```python
from build123d import *

# Parameters (mm, degrees)
F1_DEPTH = 10
F2_START = 6.1
F2_DEPTH = 3.9


with BuildPart() as f1:
    # F0 (on Front) → F1 (new body)
    with BuildSketch(Plane.XZ):
        with BuildLine():
            ThreePointArc((-36.2228804372, 67.6292184035), (-37.698913152, 69.3123111398), (-39.8481115853, 69.9387453565))
            Line((-39.8481115853, 69.9387453565), (-154.2675887644, 69.9387453565))
            Line((-154.2675887644, 69.9387453565), (-174, 66.5009789131))
            Line((-174, 66.5009789131), (-165.0019578262, 27.5261763217))
            Line((-165.0019578262, 27.5261763217), (-149.4120367897, 31.1253931912))
            ThreePointArc((-149.4120367897, 31.1253931912), (-146.3925555154, 30.6201053167), (-144.6147523132, 28.1277171494))
            Line((-144.6147523132, 28.1277171494), (-132.5798709058, -24.0010813166))
            ThreePointArc((-132.5798709058, -24.0010813166), (-133.0851587803, -27.0205625909), (-135.5775469475, -28.7983657931))
            Line((-135.5775469475, -28.7983657931), (-151.1674679841, -32.3975826626))
            Line((-151.1674679841, -32.3975826626), (-142.1694258103, -71.372385254))
            Line((-142.1694258103, -71.372385254), (-122.6820245146, -66.8733641671))
            Line((-122.6820245146, -66.8733641671), (122.6820245146, -66.8733641671))
            Line((122.6820245146, -66.8733641671), (142.1694258103, -71.372385254))
            Line((142.1694258103, -71.372385254), (151.1674679841, -32.3975826626))
            Line((151.1674679841, -32.3975826626), (135.5775469475, -28.7983657931))
            ThreePointArc((135.5775469475, -28.7983657931), (133.0851587803, -27.0205625909), (132.5798709058, -24.0010813166))
            Line((132.5798709058, -24.0010813166), (144.6147523132, 28.1277171494))
            ThreePointArc((144.6147523132, 28.1277171494), (146.3925555154, 30.6201053167), (149.4120367897, 31.1253931912))
            Line((149.4120367897, 31.1253931912), (165.0019578262, 27.5261763217))
            Line((165.0019578262, 27.5261763217), (174, 66.5009789131))
            Line((174, 66.5009789131), (154.2675887644, 69.9387453565))
            Line((154.2675887644, 69.9387453565), (39.8481115853, 69.9387453565))
            ThreePointArc((39.8481115853, 69.9387453565), (37.698913152, 69.3123111398), (36.2228804372, 67.6292184035))
            Line((36.2228804372, 67.6292184035), (6.3441545093, 3.554083875))
            ThreePointArc((6.3441545093, 3.554083875), (0, -0.4875882928), (-6.3441545093, 3.554083875))
            Line((-6.3441545093, 3.554083875), (-36.2228804372, 67.6292184035))
        make_face()
        with BuildLine():
            Line((-96.7999833788, -41.9593826596), (-92.2684444436, -39.8462913509))
            Line((-92.2684444436, -39.8462913509), (-19.7638214806, -6.0368304117))
            Line((-19.7638214806, -6.0368304117), (-15.2322825455, -3.923739103))
            ThreePointArc((-15.2322825455, -3.923739103), (-1.8101294528, -8.8090033085), (-6.6953936583, -22.2311564011))
            Line((-6.6953936583, -22.2311564011), (-11.2269325935, -24.3442477098))
            Line((-11.2269325935, -24.3442477098), (-83.7315555564, -58.1537086491))
            Line((-83.7315555564, -58.1537086491), (-88.2630944916, -60.2667999578))
            ThreePointArc((-88.2630944916, -60.2667999578), (-101.6852475843, -55.3815357523), (-96.7999833788, -41.9593826596))
        make_face(mode=Mode.SUBTRACT)
        with BuildLine():
            Line((88.2630944916, -60.2667999578), (83.7315555564, -58.1537086491))
            Line((83.7315555564, -58.1537086491), (11.2269325935, -24.3442477098))
            Line((11.2269325935, -24.3442477098), (6.6953936583, -22.2311564011))
            ThreePointArc((6.6953936583, -22.2311564011), (1.8101294528, -8.8090033085), (15.2322825455, -3.923739103))
            Line((15.2322825455, -3.923739103), (19.7638214806, -6.0368304117))
            Line((19.7638214806, -6.0368304117), (92.2684444436, -39.8462913509))
            Line((92.2684444436, -39.8462913509), (96.7999833788, -41.9593826596))
            ThreePointArc((96.7999833788, -41.9593826596), (101.6852475843, -55.3815357523), (88.2630944916, -60.2667999578))
        make_face(mode=Mode.SUBTRACT)
        with BuildLine():
            ThreePointArc((-65.576829212, -14.2695895243), (-82.8528678461, -7.9816256954), (-76.5649040173, 9.2944129387))
            Line((-76.5649040173, 9.2944129387), (-67.5018261469, 13.5205955561))
            ThreePointArc((-67.5018261469, 13.5205955561), (-50.2257875128, 7.2326317272), (-56.5137513416, -10.0434069069))
            Line((-56.5137513416, -10.0434069069), (-65.576829212, -14.2695895243))
        make_face(mode=Mode.SUBTRACT)
        with BuildLine():
            Line((-40.8102109153, 39.0972973828), (-113.3148338783, 5.2878364435))
            Line((-113.3148338783, 5.2878364435), (-117.8463728135, 3.1747451348))
            ThreePointArc((-117.8463728135, 3.1747451348), (-131.2685259061, 8.0600093403), (-126.3832617006, 21.4821624329))
            Line((-126.3832617006, 21.4821624329), (-121.8517227654, 23.5952537416))
            Line((-121.8517227654, 23.5952537416), (-49.3470998025, 57.4047146809))
            Line((-49.3470998025, 57.4047146809), (-44.8155608673, 59.5178059896))
            ThreePointArc((-44.8155608673, 59.5178059896), (-31.3934077747, 54.6325417841), (-36.2786719802, 41.2103886915))
            Line((-36.2786719802, 41.2103886915), (-40.8102109153, 39.0972973828))
        make_face(mode=Mode.SUBTRACT)
        with BuildLine():
            ThreePointArc((76.5649040173, 9.2944129387), (82.8528678461, -7.9816256954), (65.576829212, -14.2695895243))
            Line((65.576829212, -14.2695895243), (56.5137513416, -10.0434069069))
            ThreePointArc((56.5137513416, -10.0434069069), (50.2257875128, 7.2326317272), (67.5018261469, 13.5205955561))
            Line((67.5018261469, 13.5205955561), (76.5649040173, 9.2944129387))
        make_face(mode=Mode.SUBTRACT)
        with BuildLine():
            Line((49.3470998025, 57.4047146809), (121.8517227654, 23.5952537416))
            Line((121.8517227654, 23.5952537416), (126.3832617006, 21.4821624329))
            ThreePointArc((126.3832617006, 21.4821624329), (131.2685259061, 8.0600093403), (117.8463728135, 3.1747451348))
            Line((117.8463728135, 3.1747451348), (113.3148338783, 5.2878364435))
            Line((113.3148338783, 5.2878364435), (40.8102109153, 39.0972973828))
            Line((40.8102109153, 39.0972973828), (36.2786719802, 41.2103886915))
            ThreePointArc((36.2786719802, 41.2103886915), (31.3934077747, 54.6325417841), (44.8155608673, 59.5178059896))
            Line((44.8155608673, 59.5178059896), (49.3470998025, 57.4047146809))
        make_face(mode=Mode.SUBTRACT)
    extrude(amount=F1_DEPTH)

    # F0 (on Front) → F2 (join)
    with BuildSketch(Plane.XZ.offset(F2_START)):
        with BuildLine():
            Line((-117.8463728135, 3.1747451348), (-113.3148338783, 5.2878364435))
            Line((-113.3148338783, 5.2878364435), (-40.8102109153, 39.0972973828))
            Line((-40.8102109153, 39.0972973828), (-36.2786719802, 41.2103886915))
            ThreePointArc((-36.2786719802, 41.2103886915), (-31.3934077747, 54.6325417841), (-44.8155608673, 59.5178059896))
            Line((-44.8155608673, 59.5178059896), (-49.3470998025, 57.4047146809))
            Line((-49.3470998025, 57.4047146809), (-121.8517227654, 23.5952537416))
            Line((-121.8517227654, 23.5952537416), (-126.3832617006, 21.4821624329))
            ThreePointArc((-126.3832617006, 21.4821624329), (-131.2685259061, 8.0600093403), (-117.8463728135, 3.1747451348))
        make_face()
        with BuildLine():
            Line((-105.984490881, 13.2298809878), (-115.0475687514, 9.0036983703))
            ThreePointArc((-115.0475687514, 9.0036983703), (-123.0211250441, 11.9058355221), (-120.1189878923, 19.8793918148))
            Line((-120.1189878923, 19.8793918148), (-111.0559100219, 24.1055744322))
            ThreePointArc((-111.0559100219, 24.1055744322), (-103.0823537293, 21.2034372804), (-105.984490881, 13.2298809878))
        make_face(mode=Mode.SUBTRACT)
        with BuildLine():
            ThreePointArc((-47.6143649294, 53.688852754), (-39.6408086367, 50.7867156023), (-42.5429457885, 42.8131593096))
            Line((-42.5429457885, 42.8131593096), (-51.6060236588, 38.5869766922))
            ThreePointArc((-51.6060236588, 38.5869766922), (-59.5795799515, 41.489113844), (-56.6774427997, 49.4626701366))
            Line((-56.6774427997, 49.4626701366), (-47.6143649294, 53.688852754))
        make_face(mode=Mode.SUBTRACT)
        with BuildLine():
            Line((-19.7638214806, -6.0368304117), (-92.2684444436, -39.8462913509))
            Line((-92.2684444436, -39.8462913509), (-96.7999833788, -41.9593826596))
            ThreePointArc((-96.7999833788, -41.9593826596), (-101.6852475843, -55.3815357523), (-88.2630944916, -60.2667999578))
            Line((-88.2630944916, -60.2667999578), (-83.7315555564, -58.1537086491))
            Line((-83.7315555564, -58.1537086491), (-11.2269325935, -24.3442477098))
            Line((-11.2269325935, -24.3442477098), (-6.6953936583, -22.2311564011))
            ThreePointArc((-6.6953936583, -22.2311564011), (-1.8101294528, -8.8090033085), (-15.2322825455, -3.923739103))
            Line((-15.2322825455, -3.923739103), (-19.7638214806, -6.0368304117))
        make_face()
        with BuildLine():
            ThreePointArc((-85.4642904296, -54.4378467222), (-93.4378467222, -51.5357095704), (-90.5357095704, -43.5621532778))
            Line((-90.5357095704, -43.5621532778), (-81.4726317001, -39.3359706604))
            ThreePointArc((-81.4726317001, -39.3359706604), (-73.4990754074, -42.2381078121), (-76.4012125592, -50.2116641048))
            Line((-76.4012125592, -50.2116641048), (-85.4642904296, -54.4378467222))
        make_face(mode=Mode.SUBTRACT)
        with BuildLine():
            Line((-12.9596674666, -20.628385783), (-22.022745337, -24.8545684004))
            ThreePointArc((-22.022745337, -24.8545684004), (-29.9963016297, -21.9524312486), (-27.0941644779, -13.9788749559))
            Line((-27.0941644779, -13.9788749559), (-18.0310866075, -9.7526923385))
            ThreePointArc((-18.0310866075, -9.7526923385), (-10.0575303148, -12.6548294903), (-12.9596674666, -20.628385783))
        make_face(mode=Mode.SUBTRACT)
        with BuildLine():
            Line((126.3832617006, 21.4821624329), (121.8517227654, 23.5952537416))
            Line((121.8517227654, 23.5952537416), (49.3470998025, 57.4047146809))
            Line((49.3470998025, 57.4047146809), (44.8155608673, 59.5178059896))
            ThreePointArc((44.8155608673, 59.5178059896), (31.3934077747, 54.6325417841), (36.2786719802, 41.2103886915))
            Line((36.2786719802, 41.2103886915), (40.8102109153, 39.0972973828))
            Line((40.8102109153, 39.0972973828), (113.3148338783, 5.2878364435))
            Line((113.3148338783, 5.2878364435), (117.8463728135, 3.1747451348))
            ThreePointArc((117.8463728135, 3.1747451348), (131.2685259061, 8.0600093403), (126.3832617006, 21.4821624329))
        make_face()
        with BuildLine():
            ThreePointArc((120.1189878923, 19.8793918148), (123.0211250441, 11.9058355221), (115.0475687514, 9.0036983703))
            Line((115.0475687514, 9.0036983703), (105.984490881, 13.2298809878))
            ThreePointArc((105.984490881, 13.2298809878), (103.0823537293, 21.2034372804), (111.0559100219, 24.1055744322))
            Line((111.0559100219, 24.1055744322), (120.1189878923, 19.8793918148))
        make_face(mode=Mode.SUBTRACT)
        with BuildLine():
            ThreePointArc((42.5429457885, 42.8131593096), (39.6408086367, 50.7867156023), (47.6143649294, 53.688852754))
            Line((47.6143649294, 53.688852754), (56.6774427997, 49.4626701366))
            ThreePointArc((56.6774427997, 49.4626701366), (59.5795799515, 41.489113844), (51.6060236588, 38.5869766922))
            Line((51.6060236588, 38.5869766922), (42.5429457885, 42.8131593096))
        make_face(mode=Mode.SUBTRACT)
        with BuildLine():
            Line((11.2269325935, -24.3442477098), (83.7315555564, -58.1537086491))
            Line((83.7315555564, -58.1537086491), (88.2630944916, -60.2667999578))
            ThreePointArc((88.2630944916, -60.2667999578), (101.6852475843, -55.3815357523), (96.7999833788, -41.9593826596))
            Line((96.7999833788, -41.9593826596), (92.2684444436, -39.8462913509))
            Line((92.2684444436, -39.8462913509), (19.7638214806, -6.0368304117))
            Line((19.7638214806, -6.0368304117), (15.2322825455, -3.923739103))
            ThreePointArc((15.2322825455, -3.923739103), (1.8101294528, -8.8090033085), (6.6953936583, -22.2311564011))
            Line((6.6953936583, -22.2311564011), (11.2269325935, -24.3442477098))
        make_face()
        with BuildLine():
            ThreePointArc((90.5357095704, -43.5621532778), (93.4378467222, -51.5357095704), (85.4642904296, -54.4378467222))
            Line((85.4642904296, -54.4378467222), (76.4012125592, -50.2116641048))
            ThreePointArc((76.4012125592, -50.2116641048), (73.4990754074, -42.2381078121), (81.4726317001, -39.3359706604))
            Line((81.4726317001, -39.3359706604), (90.5357095704, -43.5621532778))
        make_face(mode=Mode.SUBTRACT)
        with BuildLine():
            ThreePointArc((12.9596674666, -20.628385783), (10.0575303148, -12.6548294903), (18.0310866075, -9.7526923385))
            Line((18.0310866075, -9.7526923385), (27.0941644779, -13.9788749559))
            ThreePointArc((27.0941644779, -13.9788749559), (29.9963016297, -21.9524312486), (22.022745337, -24.8545684004))
            Line((22.022745337, -24.8545684004), (12.9596674666, -20.628385783))
        make_face(mode=Mode.SUBTRACT)
    extrude(amount=F2_DEPTH)


solid = f1.part
```
For this review, take the finished solid that the model builds, in its own axes (mm). A direction names the side the tool comes from. Coordinates: 2 decimals unless noted, no trailing zeros. Answer in a Markdown table with one row per item. Add a question column.
Q1. For probe 1 along X at (y, z) = (-1.5, -13); probe 2 along X at (y, z) = (-5.25, 16); probe 3 along Z at (x, y) = (-56.5, -0.75), list the stretches that pass through material, from the lowest coordinate up.
Q2. Tool access review of faces 1 (the flat face through (61.109, -4.93, -12.186)), 2 (the flat face through (98, -5, 69.939)), 3 (the flat face through (-52, -6.1, -34)): name each direction out of +Z, -Z, +X, -X, +Y, -Y from which nothing blocks a thin tool from reaching the whole face with its end or side.
Q3. For P1, Ø5, axis at x = -99.5, y = -5, coming from the -Z side; P2, Ø2, axis at x = 72, z = 26.5, coming from the +Y side; P3, Ø2, axis at y = -2, z = -41.5, coming from the +X side, all flat-tipped, find the tip position at first contact; note any pin that passes through.
Q4. Draft analysis for pull direction Z (two halves, no side actions). For faces 4 (the flat face through (-163.996, -4.93, 68.244)), 5 (the cylindrical face through (31.3, -3.01, 54.43)), 6 (the flat face through (-2, -10, -15)), state which applies: +Z half, -Z half, draft (parallel to the pull), parting line (faces both ways), or undercut.
Q5. We need section A-A, the plane y = -4.5. Count the separate pieces of the cut face and the enclosed holes in it, and give its area (3 significant figures).
Answer list:
| question | item | result |
|---|---|---|
| 1 | probe 1 | x = -135.12 to -78.72, -62.85 to -34.7, -0.86 to 0.86, 34.7 to 62.85, 78.72 to 135.12 |
| 1 | probe 2 | x = -141.81 to -131.52, -90.34 to -12.15, 12.15 to 90.34, 131.52 to 141.81 |
| 1 | probe 3 | z = -66.87 to -45.46, -23.17 to -10.04, 13.51 to 31.78, 54.07 to 69.94 |
| 2 | face 1 | +Y, -Y |
| 2 | face 2 | +Z, +X, -X, +Y, -Y |
| 2 | face 3 | +Y |
| 3 | P1 | stops at z = -66.87 |
| 3 | P2 | stops at y = -6.1 |
| 3 | P3 | stops at x = 149.3 |
| 4 | face 4 | +Z half |
| 4 | face 5 | undercut |
| 4 | face 6 | draft |
| 5 | separate pieces | 1 |
| 5 | enclosed holes | 6 |
| 5 | area | 28,000 mm2 |
